from build123d import *

# Parameters (mm, degrees)
F1_DEPTH = 80
F2_R     = 5
F4_D     = 50


with BuildPart() as f1:
    # F0 (on Top) → F1 (new body)
    with BuildSketch(Plane.XY):
        Polygon((-56.56068, -18.37711), (9.596914, -18.37711), (9.596914, 14.497496), (9.596914, 28.382421), (-56.56068, 28.382421), align=None)
        Polygon((9.596914, 14.497496), (9.596914, -18.37711), (9.596914, -62.686369), (75.346142, -62.686369), (75.346142, 14.497496), align=None)
    extrude(amount=F1_DEPTH)

    # F2
    f2_edges = [f1.edges().sort_by_distance(p)[0] for p in [
        (9.596914, 14.497496, 40),
        (9.596914, -18.37711, 40),
        (-56.56068, -18.37711, 40),
        (-56.56068, 28.382421, 40),
        (9.596914, 28.382421, 40),
        (75.346142, 14.497496, 40),
        (75.346142, -62.686369, 40),
        (9.596914, -62.686369, 40),
    ]]
    fillet(f2_edges, radius=F2_R)

    # F4 (through all)
    with Locations(Plane.XY.offset(80)):
        with Locations((45.840353, -26.656464)):
            Hole(F4_D / 2)


solid = f1.part
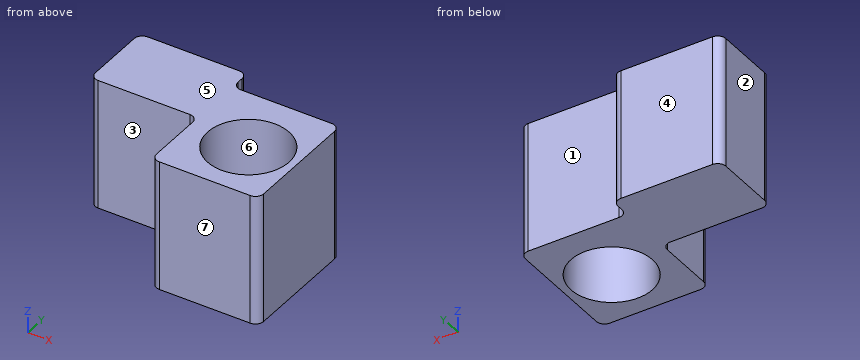
Work out the finished part from the listing and answer in its coordinate system (mm). Face numbers are marked on the shaded views. A direction names the side the tool comes from. Coordinates: 2 decimals unless noted, no trailing zeros. Write each loop counter-clockwise with the first axis right and the second up, starting at its lowest first coordinate (ties: lowest second). Pieces come first, ordered by that corner, then holes. Notation, with made-up numbers: M 14.5,8.5 L 64.5,8.5 A21 cw 64.5,21.5 Z; hole C 86,24.5 d9. An arc over 180 degrees is marked long. Answer as CSV lines item,"result". Start each with the question number.
Item 1: Section B-B on y = -39.5 is taken. Write down the section's boundary in (x, z).
Item 2: Section A-A on x = 54 is taken. Write down the section's boundary in (y, z).
Item 3: Determine the mould class of the marked faces 4, 5, 6 and 7 for opening direction Y: released by +Y, released by -Y, zero draft, split by the parting line, or undercut.
Item 4: Section D-D on x = -47.5 is taken. Write down the section's boundary in (y, z).
Item 5: Section C-C on z = 36.5 is taken. Write down the section's boundary in (x, y).
Item 6: Consider L1, parallel to X at y = -26.5, z = 28; L2, parallel to X at y = -52, z = 50; L3, parallel to Y at x = 40, z = 49.5. Determine where each line is inside the solid, lowest interval first.
Item 7: A tool of negligible diameter and unlimited length cuts with its end or side. For the marked faces 1, 2 and 3, from which of +Z, -Z, +X, -X, +Y, -Y can it reach the whole face along a straight path? Write none if from no direction.
Item 8: Flat-ended cylindrical pins translate along their axes: P1, Ø10, axis at y = -31, z = 30.5, coming from the -X side; P2, Ø1.2, axis at y = 22, z = 24.5, coming from the +X side. Find the tip coordinate at first contact, or state that the pin passes through.
Checks:
1,outline,"M 9.6,0 L 24.39,0 L 24.39,80 L 9.6,80 Z; M 67.29,0 L 75.35,0 L 75.35,80 L 67.29,80 Z"
2,outline,"M -62.69,0 L -50.29,0 L -50.29,80 L -62.69,80 Z; M -3.03,0 L 14.5,0 L 14.5,80 L -3.03,80 Z"
3,face 4,"released by +Y"
3,face 5,"zero draft"
3,face 6,"undercut"
3,face 7,"released by -Y"
4,outline,"M -18.38,0 L 28.38,0 L 28.38,80 L -18.38,80 Z"
5,outline,"M -56.56,-13.38 A5 ccw -51.56,-18.38 L 4.6,-18.38 A5 cw 9.6,-23.38 L 9.6,-57.69 A5 ccw 14.6,-62.69 L 70.35,-62.69 A5 ccw 75.35,-57.69 L 75.35,9.5 A5 ccw 70.35,14.5 L 14.6,14.5 A5 cw 9.6,19.5 L 9.6,23.38 A5 ccw 4.6,28.38 L -51.56,28.38 A5 ccw -56.56,23.38 Z; hole C 45.84,-26.66 d50"
6,L1,"x = 9.6 to 20.84, 70.84 to 75.35"
6,L2,"x = 9.6 to 75.35"
6,L3,"y = -62.69 to -50.96, -2.35 to 14.5"
7,face 1,"+Z, -Z, +X, +Y"
7,face 2,"+Z, -Z, -X, +Y, -Y"
7,face 3,"+Z, -Z, -X, -Y"
8,P1,"stops at x = 9.6"
8,P2,"stops at x = 9.6"
